from build123d import *

# Parameters (mm, degrees)
SKETCH_1_W               = 48
SKETCH_1_H               = 116
EXTRUDE_1_DEPTH          = 2
CUT_EXTRUDE_1_DEPTH      = 63.801273872
EXTRUDE_4_DEPTH          = 2
FILLET_2_R               = 2
SKETCH_7_R               = 1.6
EXTRUDE_5_DEPTH          = 2
PATTERN_LINEAR_1_COUNT   = 2
PATTERN_LINEAR_1_PITCH   = 70
MIRROR_1_COPY_1_SKETCH_R = 1.6
MIRROR_1_COPY_1_DEPTH    = 2
FILLET_4_R               = 3
FILLET_5_R               = 3
SKETCH_8_R               = 1.6
EXTRUDE_6_DEPTH          = 2
FILLET_6_R               = 3


with BuildPart() as part:
    # 草图1 → 凸台-拉伸1 (new body)
    with BuildSketch(Plane.XY):
        Rectangle(SKETCH_1_W, SKETCH_1_H)
        with BuildLine():
            Line((-19, -32), (-19, -52))
            ThreePointArc((-19, -52), (-20.1, -53.1), (-21.2, -52))
            Line((-21.2, -52), (-21.2, -32))
            ThreePointArc((-21.2, -32), (-20.1, -30.9), (-19, -32))
        make_face(mode=Mode.SUBTRACT)
        with BuildLine():
            Line((19, -32), (19, -52))
            ThreePointArc((19, -52), (20.1, -53.1), (21.2, -52))
            Line((21.2, -52), (21.2, -32))
            ThreePointArc((21.2, -32), (20.1, -30.9), (19, -32))
        make_face(mode=Mode.SUBTRACT)
        with BuildLine():
            Line((-19, 13), (-19, -7))
            ThreePointArc((-19, -7), (-20.1, -8.1), (-21.2, -7))
            Line((-21.2, -7), (-21.2, 13))
            ThreePointArc((-21.2, 13), (-20.1, 14.1), (-19, 13))
        make_face(mode=Mode.SUBTRACT)
        with BuildLine():
            Line((19, 13), (19, -7))
            ThreePointArc((19, -7), (20.1, -8.1), (21.2, -7))
            Line((21.2, -7), (21.2, 13))
            ThreePointArc((21.2, 13), (20.1, 14.1), (19, 13))
        make_face(mode=Mode.SUBTRACT)
    extrude(amount=EXTRUDE_1_DEPTH)

    # 草图3 → 切除-拉伸1 (cut, through all)
    with BuildSketch(Plane.XY.offset(2)):
        with BuildLine():
            Line((12.342439932, 19), (-14.102439932, 19))
            ThreePointArc((-14.102439932, 19), (-15.77739582, 18.092942254), (-15.933069997, 16.194522771))
            Line((-15.933069997, 16.194522771), (-2.710630065, -13.856477074))
            ThreePointArc((-2.710630065, -13.856477074), (-0.88, -15.050999845), (0.950630065, -13.856477074))
            Line((0.950630065, -13.856477074), (14.173069997, 16.194522771))
            ThreePointArc((14.173069997, 16.194522771), (14.01739582, 18.092942254), (12.342439932, 19))
        make_face()
        with BuildLine():
            Line((15.62, 5.0055453), (15.62, -46.0055453))
            ThreePointArc((15.62, -46.0055453), (14.031545787, -47.962744846), (11.789369935, -46.811022528))
            Line((11.789369935, -46.811022528), (0.566930003, -21.305477229))
            ThreePointArc((0.566930003, -21.305477229), (0.397560068, -20.5), (0.566930003, -19.694522771))
            Line((0.566930003, -19.694522771), (11.789369935, 5.811022528))
            ThreePointArc((11.789369935, 5.811022528), (14.031545787, 6.962744846), (15.62, 5.0055453))
        make_face()
        with BuildLine():
            Line((10.582439932, -56), (-12.342439932, -56))
            ThreePointArc((-12.342439932, -56), (-14.01739582, -55.092942254), (-14.173069997, -53.194522771))
            Line((-14.173069997, -53.194522771), (-2.710630065, -27.143522926))
            ThreePointArc((-2.710630065, -27.143522926), (-0.88, -25.949000155), (0.950630065, -27.143522926))
            Line((0.950630065, -27.143522926), (12.413069997, -53.194522771))
            ThreePointArc((12.413069997, -53.194522771), (12.25739582, -55.092942254), (10.582439932, -56))
        make_face()
        with BuildLine():
            Line((-17.38, 5.0055453), (-17.38, -46.0055453))
            ThreePointArc((-17.38, -46.0055453), (-15.791545787, -47.962744846), (-13.549369935, -46.811022528))
            Line((-13.549369935, -46.811022528), (-2.326930003, -21.305477229))
            ThreePointArc((-2.326930003, -21.305477229), (-2.157560068, -20.5), (-2.326930003, -19.694522771))
            Line((-2.326930003, -19.694522771), (-13.549369935, 5.811022528))
            ThreePointArc((-13.549369935, 5.811022528), (-15.791545787, 6.962744846), (-17.38, 5.0055453))
        make_face()
        with BuildLine():
            Line((10.720058136, 56), (-12.480058136, 56))
            ThreePointArc((-12.480058136, 56), (-14.332624, 54.753657562), (-13.876258409, 52.567999721))
            Line((-13.876258409, 52.567999721), (-2.276200272, 41.257943038))
            ThreePointArc((-2.276200272, 41.257943038), (-0.88, 40.689943317), (0.516200272, 41.257943038))
            Line((0.516200272, 41.257943038), (12.116258409, 52.567999721))
            ThreePointArc((12.116258409, 52.567999721), (12.572624, 54.753657562), (10.720058136, 56))
        make_face()
        with BuildLine():
            Line((19.12, 51.860056683), (19.12, 25.139943317))
            ThreePointArc((19.12, 25.139943317), (17.897045512, 23.297065059), (15.723799728, 23.707943038))
            Line((15.723799728, 23.707943038), (2.021177489, 37.067999721))
            ThreePointArc((2.021177489, 37.067999721), (1.417377761, 38.5), (2.021177489, 39.932000279))
            Line((2.021177489, 39.932000279), (15.723799728, 53.292056962))
            ThreePointArc((15.723799728, 53.292056962), (17.897045512, 53.702934941), (19.12, 51.860056683))
        make_face()
        with BuildLine():
            Line((10.720058136, 21), (-12.480058136, 21))
            ThreePointArc((-12.480058136, 21), (-14.332624, 22.246342438), (-13.876258409, 24.432000279))
            Line((-13.876258409, 24.432000279), (-2.276200272, 35.742056962))
            ThreePointArc((-2.276200272, 35.742056962), (-0.88, 36.310056683), (0.516200272, 35.742056962))
            Line((0.516200272, 35.742056962), (12.116258409, 24.432000279))
            ThreePointArc((12.116258409, 24.432000279), (12.572624, 22.246342438), (10.720058136, 21))
        make_face()
        with BuildLine():
            Line((-20.88, 51.860056683), (-20.88, 25.139943317))
            ThreePointArc((-20.88, 25.139943317), (-19.657045512, 23.297065059), (-17.483799728, 23.707943038))
            Line((-17.483799728, 23.707943038), (-3.781177489, 37.067999721))
            ThreePointArc((-3.781177489, 37.067999721), (-3.177377761, 38.5), (-3.781177489, 39.932000279))
            Line((-3.781177489, 39.932000279), (-17.483799728, 53.292056962))
            ThreePointArc((-17.483799728, 53.292056962), (-19.657045512, 53.702934941), (-20.88, 51.860056683))
        make_face()
    extrude(amount=-CUT_EXTRUDE_1_DEPTH, mode=Mode.SUBTRACT)

    # 草图6 → 凸台-拉伸4 (add)
    with BuildSketch(Plane(origin=(0, 0, 0), x_dir=(-1, 0, 0), z_dir=(0, 0, -1))):
        Polygon((-10.149479977, -48.05), (11.909479977, -48.05), (11.029479977, -46.05), (-9.269479977, -46.05), align=None)
    extrude(amount=-EXTRUDE_4_DEPTH)

    # 圆角2
    fillet_2_edges = [part.edges().sort_by_distance(p)[0] for p in [
        (10.149479977, -48.05, 1),
        (9.269479977, -46.05, 1),
        (-11.029479977, -46.05, 1),
        (-11.909479977, -48.05, 1),
    ]]
    fillet(fillet_2_edges, radius=FILLET_2_R)

    # 草图7 → 凸台-拉伸5 (add)
    with BuildSketch(Plane(origin=(0, 0, 0), x_dir=(-1, 0, 0), z_dir=(0, 0, -1))):
        with BuildLine():
            Line((24, -35.8), (34, -35.8))
            ThreePointArc((34, -35.8), (38, -31.8), (34, -27.8))
            Line((34, -27.8), (24, -27.8))
            Line((24, -27.8), (24, -35.8))
        make_face()
        with Locations((34, -31.8)):
            Circle(SKETCH_7_R, mode=Mode.SUBTRACT)
    extrude_5 = extrude(amount=-EXTRUDE_5_DEPTH)

    # 阵列(线性)1: 凸台-拉伸5 ×2
    with Locations(*[(0, i * PATTERN_LINEAR_1_PITCH, 0) for i in range(1, PATTERN_LINEAR_1_COUNT)]):
        add(extrude_5)

    # 镜向1: 凸台-拉伸5 across plane
    add(extrude_5.mirror(Plane(origin=(0, 0, 0), x_dir=(0, 0, 1), z_dir=(1, 0, 0))))

    # 镜向1 copy 1 sketch → 镜向1 copy 1 (add)
    with BuildSketch(Plane(origin=(0, 70, 0), x_dir=(1, 0, 0), z_dir=(0, 0, -1))):
        with BuildLine():
            Line((24, 35.8), (34, 35.8))
            ThreePointArc((34, 35.8), (38, 31.8), (34, 27.8))
            Line((34, 27.8), (24, 27.8))
            Line((24, 27.8), (24, 35.8))
        make_face()
        with Locations((34, 31.8)):
            Circle(MIRROR_1_COPY_1_SKETCH_R, mode=Mode.SUBTRACT)
    extrude(amount=-MIRROR_1_COPY_1_DEPTH)

    # 圆角4
    fillet_4_edges = [part.edges().sort_by_distance(p)[0] for p in [
        (-24, 58, 1),
        (24, 58, 1),
        (24, -58, 1),
        (-24, -58, 1),
    ]]
    fillet(fillet_4_edges, radius=FILLET_4_R)

    # 圆角5
    fillet_5_edges = [part.edges().sort_by_distance(p)[0] for p in [
        (-24, -35.8, 1),
        (-24, -27.8, 1),
        (-24, 34.2, 1),
        (-24, 42.2, 1),
        (24, -27.8, 1),
        (24, -35.8, 1),
        (24, 42.2, 1),
        (24, 34.2, 1),
    ]]
    fillet(fillet_5_edges, radius=FILLET_5_R)

    # 草图8 → 凸台-拉伸6 (add)
    # profile 1 of 2: a face of its own
    with BuildSketch(Plane.XY.offset(2)):
        with BuildLine():
            Line((-34, -1.8), (-24, -1.8))
            Line((-24, -1.8), (-24, 8.2))
            Line((-24, 8.2), (-34, 8.2))
            ThreePointArc((-34, 8.2), (-39, 3.2), (-34, -1.8))
        make_face()
        with Locations((-34, 3.2)):
            Circle(SKETCH_8_R, mode=Mode.SUBTRACT)
    # profile 2 of 2: a face of its own
    with BuildSketch(Plane.XY.offset(2)):
        with BuildLine():
            Line((24, 8.2), (24, -1.8))
            Line((24, -1.8), (34, -1.8))
            ThreePointArc((34, -1.8), (39, 3.2), (34, 8.2))
            Line((34, 8.2), (24, 8.2))
        make_face()
        with Locations(Location((34, 3.2, 0), (0, 0, 180))):
            Circle(SKETCH_8_R, mode=Mode.SUBTRACT)
    extrude(amount=-EXTRUDE_6_DEPTH)

    # 圆角6
    fillet_6_edges = [part.edges().sort_by_distance(p)[0] for p in [
        (-24, 8.2, 1),
        (-24, -1.8, 1),
        (24, -1.8, 1),
        (24, 8.2, 1),
    ]]
    fillet(fillet_6_edges, radius=FILLET_6_R)


solid = part.part
Check sheet for the modelled part. Datum: model origin and axes. Units: mm. A direction names the side the tool comes from. Give positions to 0.01 mm unless a question says otherwise; leave off trailing zeros. Loops run counter-clockwise (first coordinate to the right, second up) from the corner with the lowest first, then second, coordinate; pieces in that order, holes last. Notation, with made-up numbers: M 18.25,53 L 50.25,53 A28 ccw 50.25,92 Z; hole C -33.5,32.25 d7. An arc over 180 degrees is marked long. Answer as a JSON object with one key per item and string values. Group by question number.
Q1. Access from +Z, -Z, +X, -X, +Y, -Y to the whole of each face (thin tool, end or side, straight path). Record for faces 1 (the cylindrical face through (-24.9, -26.94, 1.01)), 2 (the cylindrical face through (24.86, -2.7, 0.99)), 3 (the flat face through (6.2, 46.8, 1)).
Q2. Cross-section at B-B on x = -31. Record the cut outline in (y, z), then the cut area to 3 significant figures.
Q3. Cross-section at D-D on x = 3.5. Give the number of separate pieces and of enclosed holes in the cut face, then the cut area to 3 significant figures.
Q4. Material ranges on line 1 along Y through (x, z) = (34, 0.4); line 2 along X through (y, z) = (38.2, 0.5); line 3 along Y through (x, z) = (17, 0.6), recorded low to high. Write a range as [from, to].
Q5. Cross-section at C-C on y = -3. Record the cut outline in (x, z).
Q6. Cross-section at A-A on y = 38.2. Record the cut outline in (x, z).
Q7. Go/stop test with flat-tipped pins: P1, Ø6, axis at x = -8, y = 7.5, coming from the -Z side; P2, Ø1, axis at y = 25, z = 0.5, coming from the +X side; P3, Ø5, axis at x = -34, y = 38.2, coming from the +Z side; P4, Ø0.6, axis at y = 5.5, z = 1.5, coming from the -X side. Record where each tip stops, or that it passes through.
Q8. Release check for a two-part mould opening along Y. For faces 4 (the flat face through (-9.414, 1.379, 1.014)), 5 (the flat face through (6.26, -34.24, 1.01)), 6 (the flat face through (6, -4, 2)), 7 (the cylindrical face through (23.14, 57.1, 1.01)) record: released by +Y, released by -Y, zero draft, split by the parting line, or undercut.
Evaluation:
{
 "1": {"face 1": "+Z, -Z, -X", "face 2": "+Z, -Z, +X", "face 3": "+Z, -Z"},
 "2": {"outline": "M -35.8,0 L -27.8,0 L -27.8,2 L -35.8,2 Z; M -1.8,0 L 8.2,0 L 8.2,2 L -1.8,2 Z; M 34.2,0 L 42.2,0 L 42.2,2 L 34.2,2 Z", "area": "52.0 mm2"},
 "3": {"separate pieces": "8", "enclosed holes": "0", "area": "47.0 mm2"},
 "4": {"line 1": "y = [-35.8, -33.4], [-30.2, -27.8], [-1.8, 1.6], [4.8, 8.2], [34.2, 36.6], [39.8, 42.2]", "line 2": "x = [-38, -35.6], [-32.4, -20.88], [-3.2, 1.44], [19.12, 32.4], [35.6, 38]", "line 3": "y = [-58, 23.14], [53.86, 58]"},
 "5": {"outline": "M -24.6,0 L -21.2,0 L -21.2,2 L -24.6,2 Z; M -19,0 L -17.38,0 L -17.38,2 L -19,2 Z; M -9.67,0 L -7.49,0 L -7.49,2 L -9.67,2 Z; M 5.73,0 L 7.91,0 L 7.91,2 L 5.73,2 Z; M 15.62,0 L 19,0 L 19,2 L 15.62,2 Z; M 21.2,0 L 24.6,0 L 24.6,2 L 21.2,2 Z"},
 "6": {"outline": "M -38,0 L -35.6,0 L -35.6,2 L -38,2 Z; M -32.4,0 L -20.88,0 L -20.88,2 L -32.4,2 Z; M -3.2,0 L 1.44,0 L 1.44,2 L -3.2,2 Z; M 19.12,0 L 32.4,0 L 32.4,2 L 19.12,2 Z; M 35.6,0 L 38,0 L 38,2 L 35.6,2 Z"},
 "7": {"P1": "passes through", "P2": "stops at x = 24", "P3": "stops at z = 2", "P4": "stops at x = -38.58"},
 "8": {"face 4": "undercut", "face 5": "undercut", "face 6": "zero draft", "face 7": "released by +Y"}
}
